The figure shows three views and two pictorial views of one solid part (mm, origin at its lowest corner). Answer the questions. A direction names the side the tool comes from. Give positions to 0.01 mm unless a question says otherwise; leave off trailing zeros. Loops run counter-clockwise (first coordinate to the right, second up) from the corner with the lowest first, then second, coordinate; pieces in that order, holes last. Notation, with made-up numbers: M 73,-27 L 100,-27 A21 cw 100,-20 Z; hole C 85,80 d4. An arc over 180 degrees is marked long. One line per item, written item: value. Start each with the question number.
Q1. For the marked faces 1 and 2, determine the directions among +Z, -Z, +X, -X, +Y, -Y from which every point of the face is accessible in a straight line to the end or side of a thin tool.
Q2. Consider L1, parallel to Y at x = 13.5, z = 180.34; L2, parallel to X at y = 67, z = 140.5; L3, parallel to Z at x = 36, y = 50 (1 decimal). Determine where each line is inside the solid, lowest interval first.
Q3. A cutting plane is placed at A-A, the plane z = 180.34. Determine the outline of the cut face in (x, y), and give its area (3 significant figures).
Q4. A cutting plane is placed at C-C, the plane x = 45.5. Determine the outline of the cut face in (y, z).
Q5. A cutting plane is placed at B-B, the plane y = 50.8. Determine the outline of the cut face in (x, z).
Q6. Flat-ended cylindrical pins translate along their axes: pin 1 (4 mm diameter, centred on x = 41, y = 34, fed in from +Z); pin 2 (3 mm diameter, centred on x = 15.5, z = 182.5, fed in from +Y); pin 3 (8 mm diameter, centred on x = 34, y = 89.5, fed in from +Z). Find the tip coordinate at first contact, or state that the pin passes through.
Q7. A cutting plane is placed at D-D, the plane z = 38.1. Determine the outline of the cut face in (x, y), and give its area (3 significant figures).
Q8. The mould has two halves that part along Y. Classify the marked faces 3, 4 and 5: +Y half, -Y half, draft (parallel to the pull), parting line (faces both ways), or undercut.
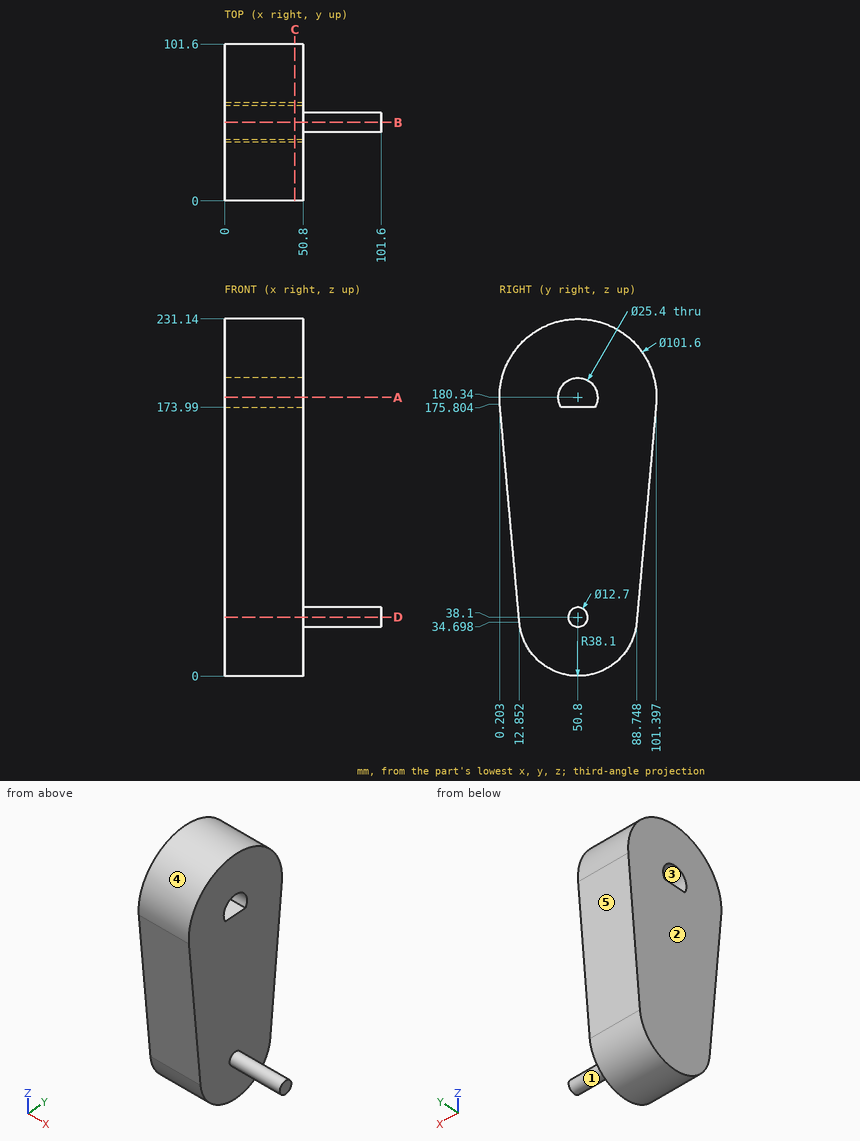
Answer block:
1. face 1: +X
1. face 2: +Z, -Z, -X, +Y, -Y
2. L1: 0 to 38.1, 63.5 to 101.6
2. L2: 0 to 50.8
2. L3: 0 to 174, 193 to 231.1
3. outline: M 0,0 L 50.8,0 L 50.8,38.1 L 0,38.1 Z; M 0,63.5 L 50.8,63.5 L 50.8,101.6 L 0,101.6 Z
3. area: 3,870 mm^2
4. outline: M 0.2,175.8 L 12.85,34.7 A38.1 ccw 88.75,34.7 L 101.4,175.8 A50.8 ccw long Z; hole M 39.8,173.99 L 61.8,173.99 A12.7 ccw long Z
5. outline: M 0,0 L 50.8,0 L 50.8,31.75 L 101.6,31.75 L 101.6,44.45 L 50.8,44.45 L 50.8,173.99 L 0,173.99 Z; M 0,193.04 L 50.8,193.04 L 50.8,231.14 L 0,231.14 Z
6. pin 1: z = 228.94
6. pin 2: y = 101.6
6. pin 3: z = 217.44
7. outline: M 0,12.55 L 50.8,12.55 L 50.8,44.45 L 101.6,44.45 L 101.6,57.15 L 50.8,57.15 L 50.8,89.05 L 0,89.05 Z
7. area: 4,530 mm^2
8. face 3: undercut
8. face 4: parting line
8. face 5: +Y half
